from build123d import *

# Parameters (mm, degrees)
SKETCH1_R                   = 8.9916
BOSS_EXTRUDE1_DEPTH         = 3.175
SKETCH2_R                   = 6.9453125
BOSS_EXTRUDE2_DEPTH         = 6.35
F_21_0_159_DIAMETER_HOLE1_D = 4.7625


with BuildPart() as part:
    # Sketch1 → Boss-Extrude1 (new body)
    with BuildSketch(Plane(origin=(0, 0, 0), x_dir=(0, 0, -1), z_dir=(1, 0, 0))):
        Circle(SKETCH1_R)
    extrude(amount=BOSS_EXTRUDE1_DEPTH)

    # Sketch2 → Boss-Extrude2 (add)
    with BuildSketch(Plane.ZY):
        with Locations(Location((0, 0, 0), (0, 0, 180))):
            Circle(SKETCH2_R)
    extrude(amount=BOSS_EXTRUDE2_DEPTH)

    # #21 (0.159) Diameter Hole1 (through all)
    with Locations(Plane.ZY.offset(6.35)):
        with Locations((0, 0)):
            Hole(F_21_0_159_DIAMETER_HOLE1_D / 2)


solid = part.part
Source: CAD feature listing. Evaluate the final solid. Frame: model axes, mm. A direction names the side the tool comes from. Give positions to 0.01 mm unless a question says otherwise; leave off trailing zeros. Write each loop counter-clockwise with the first axis right and the second up, starting at its lowest first coordinate (ties: lowest second). Pieces come first, ordered by that corner, then holes. Notation, with made-up numbers: (29, 44.5) -> (35, 44.5) arc R31 cw to (35, 75.5) -> close; hole circle Ø1 at (-20.5, 56). An arc over 180 degrees is marked (long way). Return JSON: item names as keys, results as strings. Group by question number.
1. Material intervals for line 1 (Y direction, x = -0.75, z = 0); line 2 (Y direction, x = 1.25, z = 0); line 3 (Z direction, x = -3, y = -0.25), sorted ascending. Write a range as from..to.
2. Section D-D, the plane z = -3. Output: boundary loops of the cut face in (x, y) (3 decimals), then the cut area to 3 significant figures.
3. Access query for faces 1 (the face through (-3.131, -6.886, 0.904)), 2 (the face through (3.175, -2, -2)). Directions: +Z, -Z, +X, -X, +Y, -Y. A direction counts if a zero-diameter tool reaches every point of the face in a straight line with its end or side. Return the directions, or none.
4. Mould query, pull axis Z, two halves, no side actions, for faces 3 (the face through (1.565, -3.444, -8.306)), 4 (the face through (-6.35, 0, -3)), 5 (the face through (-1.52, -1.45, 1.89)). Classes: +Z half, -Z half, draft (parallel to the pull), parting line (faces both ways), or undercut.
5. Section C-C, the plane x = -2.5. Output: boundary loops of the cut face in (y, z).
6. Section A-A, the plane z = 0. Output: boundary loops of the cut face in (x, y) (3 decimals).
7. Pin query (flat end, axial travel): pin 1 Ø1 at (x, z) = (-4, -2.5) entering from +Y; pin 2 Ø4 at (x, y) = (2, 2.5) entering from +Z; pin 3 Ø2 at (x, y) = (0.5, 4.5) entering from -Z. Return the tip coordinate at first contact, or that it passes through.
Determined:
{
 "1": {"line 1": "y = -6.95..-2.38, 2.38..6.95", "line 2": "y = -8.99..-2.38, 2.38..8.99", "line 3": "z = -6.94..-2.37, 2.37..6.94"},
 "2": {"outline": "(-6.35, -6.264) -> (0, -6.264) -> (0, -8.476) -> (3.175, -8.476) -> (3.175, 8.476) -> (0, 8.476) -> (0, 6.264) -> (-6.35, 6.264) -> close", "area": "133 mm2"},
 "3": {"face 1": "-X", "face 2": "+Z, -Z, +X, +Y, -Y"},
 "4": {"face 3": "parting line", "face 4": "draft", "face 5": "undercut"},
 "5": {"outline": "circle Ø13.89 at (0, 0); hole circle Ø4.76 at (0, 0)"},
 "6": {"outline": "(-6.35, -6.945) -> (0, -6.945) -> (0, -8.992) -> (3.175, -8.992) -> (3.175, -2.381) -> (-6.35, -2.381) -> close; (-6.35, 2.381) -> (3.175, 2.381) -> (3.175, 8.992) -> (0, 8.992) -> (0, 6.945) -> (-6.35, 6.945) -> close"},
 "7": {"pin 1": "stops at y = 6.65", "pin 2": "stops at z = 8.98", "pin 3": "stops at z = -8.28"}
}
